For this review, take the finished solid that the model builds, in its own axes (mm). Face numbers are marked on the shaded views. Round coordinates to 2 decimals unless told otherwise and drop trailing zeros. Order: outer loops, then holes, each group sorted by start corner. A loop starts at its lowest first (then second) coordinate and runs counter-clockwise, first axis right, second up. Notation, with made-up numbers: M 72.5,-3 L 77.5,-3 A18 ccw 77.5,25 Z; hole C -39.5,11.25 d6. An arc over 180 degrees is marked long. Answer in a Markdown table with one row per item. Add a question column.
```python
from build123d import *

# Parameters (mm, degrees)
ESBO_O1_W                = 37.61
ESBO_O1_H                = 19.56
BASE_DEPTH               = 3
ESPA_O_START             = 3
ESBO_O4_W                = 33.11
ESBO_O4_H                = 15.06
ESPA_O_SENSOR_DEPTH      = 1.5
RECORTE_START            = 1.5
ESBO_O5_W                = 5
ESBO_O5_H                = 10.16
RECORTE_CONECTORES_DEPTH = 23.907391831
ESBO_O6_R                = 0.75
CORTE_EXTRUS_O3_DEPTH    = 2


with BuildPart() as part:
    # Esboço1 → Base (new body)
    with BuildSketch(Plane(origin=(0, 0, 0), x_dir=(1, 0, 0), z_dir=(0, 1, 0))):
        Rectangle(ESBO_O1_W, ESBO_O1_H)
    extrude(amount=BASE_DEPTH)

    # Esboço4 → Espaço Sensor (cut)
    with BuildSketch(Plane(origin=(0, 0, 0), x_dir=(1, 0, 0), z_dir=(0, 1, 0)).offset(ESPA_O_START)):
        Rectangle(ESBO_O4_W, ESBO_O4_H)
    extrude(amount=-ESPA_O_SENSOR_DEPTH, mode=Mode.SUBTRACT)

    # Esboço5 → Recorte Conectores (cut, through all)
    with BuildSketch(Plane(origin=(0, 0, 0), x_dir=(1, 0, 0), z_dir=(0, 1, 0)).offset(RECORTE_START)):
        with Locations((-13.555, 0)):
            Rectangle(ESBO_O5_W, ESBO_O5_H)
    extrude(amount=-RECORTE_CONECTORES_DEPTH, mode=Mode.SUBTRACT)

    # Esboço6 → Corte-extrusão3 (cut)
    with BuildSketch(Plane(origin=(0, 0, 0), x_dir=(1, 0, 0), z_dir=(0, 1, 0))):
        with Locations(Location((-17.68, -8.655, 0), (0, 0, 270))):
            Circle(ESBO_O6_R)
        with Locations(Location((17.68, -8.655, 0), (0, 0, 270))):
            Circle(ESBO_O6_R)
        with Locations(Location((17.68, 8.655, 0), (0, 0, 270))):
            Circle(ESBO_O6_R)
        with Locations(Location((-17.68, 8.655, 0), (0, 0, 270))):
            Circle(ESBO_O6_R)
    extrude(amount=CORTE_EXTRUS_O3_DEPTH, mode=Mode.SUBTRACT)


solid = part.part
```
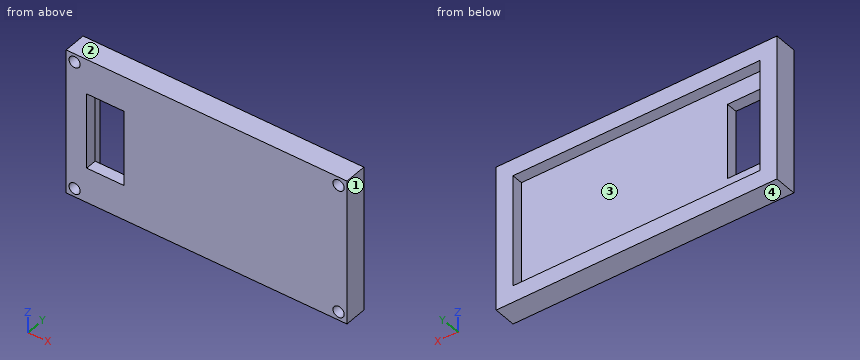
1. Clearance check with flat-ended pins moving along their axes: pin 1 Ø0.8 at (x, z) = (-17.5, 8.5) entering from -Y; pin 2 Ø8 at (x, z) = (11, 1) entering from +Y. State where each tip first meets the part, or that it passes through.
2. Consider section C-C on x = -17.68. Write out the cut boundary in (y, z) (3 decimals), plus the area to 3 significant figures.
3. Consider section D-D on x = 7. Write out the cut boundary in (y, z).
4. The part is to be moulded in two halves that separate along Z. For the marked faces 1, 2, 3 and 4, say which applies: pulls with the +Z half, pulls with the -Z half, needs draft (parallel to the pull), parting line crosses it, or undercut.
5. To check wall thickness, follow probe 1 along X at (y, z) = (2.6, 1) (3 decimals); probe 2 along X at (y, z) = (0.45, -3.75) (3 decimals); probe 3 along Z at (x, y) = (-2, 2.1). State the ranges of each line that lie inside material, in increasing order. Write a range as [from, to].
6. Consider section A-A on z = -4. Write out the cut boundary in (x, y) (3 decimals), plus the area to 3 significant figures.
7. Consider section B-B on y = 0.95. Write out the cut boundary in (x, z) (3 decimals).
Solved:
| question | item | result |
|---|---|---|
| 1 | pin 1 | stops at y = 2 |
| 1 | pin 2 | stops at y = 1.5 |
| 2 | outline | M 0,-9.78 L 3,-9.78 L 3,9.78 L 0,9.78 L 0,9.405 L 2,9.405 L 2,7.905 L 0,7.905 L 0,-7.905 L 2,-7.905 L 2,-9.405 L 0,-9.405 Z |
| 2 | area | 52.7 mm^2 |
| 3 | outline | M 0,-9.78 L 3,-9.78 L 3,-7.53 L 1.5,-7.53 L 1.5,7.53 L 3,7.53 L 3,9.78 L 0,9.78 Z |
| 4 | face 1 | needs draft |
| 4 | face 2 | pulls with the +Z half |
| 4 | face 3 | undercut |
| 4 | face 4 | pulls with the -Z half |
| 5 | probe 1 | x = [-18.805, -16.555], [16.555, 18.805] |
| 5 | probe 2 | x = [-18.805, -16.055], [-11.055, 18.805] |
| 5 | probe 3 | z = [-9.78, -7.53], [7.53, 9.78] |
| 6 | outline | M -18.805,0 L -16.055,0 L -16.055,1.5 L -16.555,1.5 L -16.555,3 L -18.805,3 Z; M -11.055,0 L 18.805,0 L 18.805,3 L 16.555,3 L 16.555,1.5 L -11.055,1.5 Z |
| 6 | area | 55.7 mm^2 |
| 7 | outline | M -18.805,-9.78 L 18.805,-9.78 L 18.805,9.78 L -18.805,9.78 Z; hole C -17.68,-8.655 d1.5; hole C -17.68,8.655 d1.5; hole M -16.055,-5.08 L -11.055,-5.08 L -11.055,5.08 L -16.055,5.08 Z; hole C 17.68,-8.655 d1.5; hole C 17.68,8.655 d1.5 |
